The model under review builds one solid part; all positions refer to its coordinate system, in mm. Face numbers are marked on the shaded views. A direction names the side the tool comes from. Round coordinates to 2 decimals unless told otherwise and drop trailing zeros. Loops run counter-clockwise (first coordinate to the right, second up) from the corner with the lowest first, then second, coordinate; pieces in that order, holes last. Notation, with made-up numbers: M 52.5,7.25 L 88.5,7.25 A9 ccw 88.5,23.25 Z; hole C 19,2.5 d6. An arc over 180 degrees is marked long. Return JSON: item names as keys, results as strings. Group by question number.
Q1. Consider section A-A (y = 4.95). State the section outline as (x, z) points.
Q2. To check wall thickness, follow line 1 along Z through (x, y) = (-1.5, 5.3); line 2 along X through (y, z) = (2.05, -0.5); line 3 along Y through (x, z) = (0.25, -0.5). State the ranges of each line that lie inside material, in increasing order.
Q3. Consider section C-C (z = 0.75). State the section outline as (x, y) points.
Q4. Clearance check with flat-ended pins moving along their axes: pin 1 Ø3 at (x, z) = (0, 0) entering from +Y; pin 2 Ø1 at (x, y) = (-0.5, 5) entering from +Z. State where each tip first meets the part, or that it passes through.
Q5. Consider section B-B (x = -1.25). State the section outline as (y, z) points, and give its area (3 significant figures).
Q6. For the marked faces 1 and 2, list the 3-axis set-ups (+Z, -Z, +X, -X, +Y, -Y) from which the entire face can be reached by the end or side of a thin tool; tool diameter is ignored.
Q7. Consider section D-D (z = 2.75). State the section outline as (x, y) points.
Q8. Draft analysis for pull direction X (two halves, no side actions). For the marked faces 3, 4 and 5, state which applies: pulls with the +X half, pulls with the -X half, needs draft (parallel to the pull), parting line crosses it, or undercut.
from build123d import *

# Parameters (mm, degrees)
BOSS_EXTRUDE1_DEPTH = 6
SKETCH2_W           = 4
SKETCH2_H           = 4
CUT_EXTRUDE1_DEPTH  = 5
FILLET1_R           = 0.25


with BuildPart() as part:
    # Sketch1 → Boss-Extrude1 (new body)
    with BuildSketch(Plane(origin=(0, 0, 0), x_dir=(1, 0, 0), z_dir=(0, 1, 0))):
        Polygon((3.214834695, -1.383776673), (2.8058031, 2.092240179), (-0.409031596, 3.476016852), (-3.214834695, 1.383776673), (-2.8058031, -2.092240179), (0.409031596, -3.476016852), align=None)
    extrude(amount=BOSS_EXTRUDE1_DEPTH)

    # Sketch2 → Cut-Extrude1 (cut)
    with BuildSketch(Plane(origin=(0, 6, 0), x_dir=(1, 0, 0), z_dir=(0, 1, 0))):
        Rectangle(SKETCH2_W, SKETCH2_H)
    extrude(amount=-CUT_EXTRUDE1_DEPTH, mode=Mode.SUBTRACT)

    # Fillet1
    # the kernel refuses this fillet: 0.25 mm, written as the material it takes off along each edge
    with BuildSketch(Plane(origin=(-2, 6, -2), x_dir=(-1, 0, 0), z_dir=(0, 0, 1)), Plane(origin=(2, 6, -2), x_dir=(0, 0, -1), z_dir=(-1, 0, 0)), Plane(origin=(-2, 6, 2), x_dir=(0, 0, 1), z_dir=(1, 0, 0)), Plane(origin=(2, 6, 2), x_dir=(1, 0, 0), z_dir=(0, 0, -1))) as fillet1_piece_1:
        with BuildLine():
            CenterArc((FILLET1_R, FILLET1_R), FILLET1_R, 180, 90)
            Line((0, FILLET1_R), (-FILLET1_R * 0.02, FILLET1_R))
            Line((-FILLET1_R * 0.02, FILLET1_R), (-FILLET1_R * 0.02, -FILLET1_R * 0.02))
            Line((-FILLET1_R * 0.02, -FILLET1_R * 0.02), (FILLET1_R, -FILLET1_R * 0.02))
            Line((FILLET1_R, -FILLET1_R * 0.02), (FILLET1_R, 0))
        make_face()
    extrude(amount=4, mode=Mode.SUBTRACT)
    with BuildSketch(Plane(origin=(2, 6, -2), x_dir=(0, 0, -1), z_dir=(-1, 0, 0))) as fillet1_piece_2a_section:
        with BuildLine():
            CenterArc((FILLET1_R, FILLET1_R), FILLET1_R, 180, 90)
            Line((0, FILLET1_R), (-FILLET1_R * 0.02, FILLET1_R))
            Line((-FILLET1_R * 0.02, FILLET1_R), (-FILLET1_R * 0.02, -FILLET1_R * 0.02))
            Line((-FILLET1_R * 0.02, -FILLET1_R * 0.02), (FILLET1_R, -FILLET1_R * 0.02))
            Line((FILLET1_R, -FILLET1_R * 0.02), (FILLET1_R, 0))
        make_face()
    fillet1_piece_2a = extrude(amount=4.625, mode=Mode.PRIVATE)
    fillet1_piece_2a = split(fillet1_piece_2a, bisect_by=Plane(origin=(-2, 5.943401221, -2.056598779), z_dir=(-1, 0, 0)), keep=Keep.TOP, mode=Mode.PRIVATE)
    with BuildSketch(Plane(origin=(-2, 6, -2.625), x_dir=(-1, 0, 0), z_dir=(0, 0, 1))) as fillet1_piece_2b_section:
        with BuildLine():
            CenterArc((FILLET1_R, FILLET1_R), FILLET1_R, 180, 90)
            Line((0, FILLET1_R), (-FILLET1_R * 0.02, FILLET1_R))
            Line((-FILLET1_R * 0.02, FILLET1_R), (-FILLET1_R * 0.02, -FILLET1_R * 0.02))
            Line((-FILLET1_R * 0.02, -FILLET1_R * 0.02), (FILLET1_R, -FILLET1_R * 0.02))
            Line((FILLET1_R, -FILLET1_R * 0.02), (FILLET1_R, 0))
        make_face()
    fillet1_piece_2b = extrude(amount=4.625, mode=Mode.PRIVATE)
    fillet1_piece_2b = split(fillet1_piece_2b, bisect_by=Plane(origin=(-2.056598779, 5.943401221, -2), z_dir=(0, 0, -1)), keep=Keep.TOP, mode=Mode.PRIVATE)
    fillet1_piece_2 = fillet1_piece_2a & fillet1_piece_2b
    add(fillet1_piece_2, mode=Mode.SUBTRACT)
    with BuildSketch(Plane(origin=(-2.625, 6, 2), x_dir=(0, 0, 1), z_dir=(1, 0, 0))) as fillet1_piece_3a_section:
        with BuildLine():
            CenterArc((FILLET1_R, FILLET1_R), FILLET1_R, 180, 90)
            Line((0, FILLET1_R), (-FILLET1_R * 0.02, FILLET1_R))
            Line((-FILLET1_R * 0.02, FILLET1_R), (-FILLET1_R * 0.02, -FILLET1_R * 0.02))
            Line((-FILLET1_R * 0.02, -FILLET1_R * 0.02), (FILLET1_R, -FILLET1_R * 0.02))
            Line((FILLET1_R, -FILLET1_R * 0.02), (FILLET1_R, 0))
        make_face()
    fillet1_piece_3a = extrude(amount=4.625, mode=Mode.PRIVATE)
    fillet1_piece_3a = split(fillet1_piece_3a, bisect_by=Plane(origin=(-2, 5.943401221, 2.056598779), z_dir=(-1, 0, 0)), keep=Keep.TOP, mode=Mode.PRIVATE)
    with BuildSketch(Plane(origin=(-2, 6, -2), x_dir=(-1, 0, 0), z_dir=(0, 0, 1))) as fillet1_piece_3b_section:
        with BuildLine():
            CenterArc((FILLET1_R, FILLET1_R), FILLET1_R, 180, 90)
            Line((0, FILLET1_R), (-FILLET1_R * 0.02, FILLET1_R))
            Line((-FILLET1_R * 0.02, FILLET1_R), (-FILLET1_R * 0.02, -FILLET1_R * 0.02))
            Line((-FILLET1_R * 0.02, -FILLET1_R * 0.02), (FILLET1_R, -FILLET1_R * 0.02))
            Line((FILLET1_R, -FILLET1_R * 0.02), (FILLET1_R, 0))
        make_face()
    fillet1_piece_3b = extrude(amount=4.625, mode=Mode.PRIVATE)
    fillet1_piece_3b = split(fillet1_piece_3b, bisect_by=Plane(origin=(-2.056598779, 5.943401221, 2), z_dir=(0, 0, 1)), keep=Keep.TOP, mode=Mode.PRIVATE)
    fillet1_piece_3 = fillet1_piece_3a & fillet1_piece_3b
    add(fillet1_piece_3, mode=Mode.SUBTRACT)
    with BuildSketch(Plane(origin=(2, 6, 2), x_dir=(1, 0, 0), z_dir=(0, 0, -1))) as fillet1_piece_4a_section:
        with BuildLine():
            CenterArc((FILLET1_R, FILLET1_R), FILLET1_R, 180, 90)
            Line((0, FILLET1_R), (-FILLET1_R * 0.02, FILLET1_R))
            Line((-FILLET1_R * 0.02, FILLET1_R), (-FILLET1_R * 0.02, -FILLET1_R * 0.02))
            Line((-FILLET1_R * 0.02, -FILLET1_R * 0.02), (FILLET1_R, -FILLET1_R * 0.02))
            Line((FILLET1_R, -FILLET1_R * 0.02), (FILLET1_R, 0))
        make_face()
    fillet1_piece_4a = extrude(amount=4.625, mode=Mode.PRIVATE)
    fillet1_piece_4a = split(fillet1_piece_4a, bisect_by=Plane(origin=(2.056598779, 5.943401221, -2), z_dir=(0, 0, -1)), keep=Keep.TOP, mode=Mode.PRIVATE)
    with BuildSketch(Plane(origin=(2.625, 6, -2), x_dir=(0, 0, -1), z_dir=(-1, 0, 0))) as fillet1_piece_4b_section:
        with BuildLine():
            CenterArc((FILLET1_R, FILLET1_R), FILLET1_R, 180, 90)
            Line((0, FILLET1_R), (-FILLET1_R * 0.02, FILLET1_R))
            Line((-FILLET1_R * 0.02, FILLET1_R), (-FILLET1_R * 0.02, -FILLET1_R * 0.02))
            Line((-FILLET1_R * 0.02, -FILLET1_R * 0.02), (FILLET1_R, -FILLET1_R * 0.02))
            Line((FILLET1_R, -FILLET1_R * 0.02), (FILLET1_R, 0))
        make_face()
    fillet1_piece_4b = extrude(amount=4.625, mode=Mode.PRIVATE)
    fillet1_piece_4b = split(fillet1_piece_4b, bisect_by=Plane(origin=(2, 5.943401221, -2.056598779), z_dir=(1, 0, 0)), keep=Keep.TOP, mode=Mode.PRIVATE)
    fillet1_piece_4 = fillet1_piece_4a & fillet1_piece_4b
    add(fillet1_piece_4, mode=Mode.SUBTRACT)
    with BuildSketch(Plane(origin=(-2, 6, 2), x_dir=(0, 0, 1), z_dir=(1, 0, 0))) as fillet1_piece_5a_section:
        with BuildLine():
            CenterArc((FILLET1_R, FILLET1_R), FILLET1_R, 180, 90)
            Line((0, FILLET1_R), (-FILLET1_R * 0.02, FILLET1_R))
            Line((-FILLET1_R * 0.02, FILLET1_R), (-FILLET1_R * 0.02, -FILLET1_R * 0.02))
            Line((-FILLET1_R * 0.02, -FILLET1_R * 0.02), (FILLET1_R, -FILLET1_R * 0.02))
            Line((FILLET1_R, -FILLET1_R * 0.02), (FILLET1_R, 0))
        make_face()
    fillet1_piece_5a = extrude(amount=4.625, mode=Mode.PRIVATE)
    fillet1_piece_5a = split(fillet1_piece_5a, bisect_by=Plane(origin=(2, 5.943401221, 2.056598779), z_dir=(1, 0, 0)), keep=Keep.TOP, mode=Mode.PRIVATE)
    with BuildSketch(Plane(origin=(2, 6, 2.625), x_dir=(1, 0, 0), z_dir=(0, 0, -1))) as fillet1_piece_5b_section:
        with BuildLine():
            CenterArc((FILLET1_R, FILLET1_R), FILLET1_R, 180, 90)
            Line((0, FILLET1_R), (-FILLET1_R * 0.02, FILLET1_R))
            Line((-FILLET1_R * 0.02, FILLET1_R), (-FILLET1_R * 0.02, -FILLET1_R * 0.02))
            Line((-FILLET1_R * 0.02, -FILLET1_R * 0.02), (FILLET1_R, -FILLET1_R * 0.02))
            Line((FILLET1_R, -FILLET1_R * 0.02), (FILLET1_R, 0))
        make_face()
    fillet1_piece_5b = extrude(amount=4.625, mode=Mode.PRIVATE)
    fillet1_piece_5b = split(fillet1_piece_5b, bisect_by=Plane(origin=(2.056598779, 5.943401221, 2), z_dir=(0, 0, 1)), keep=Keep.TOP, mode=Mode.PRIVATE)
    fillet1_piece_5 = fillet1_piece_5a & fillet1_piece_5b
    add(fillet1_piece_5, mode=Mode.SUBTRACT)


solid = part.part
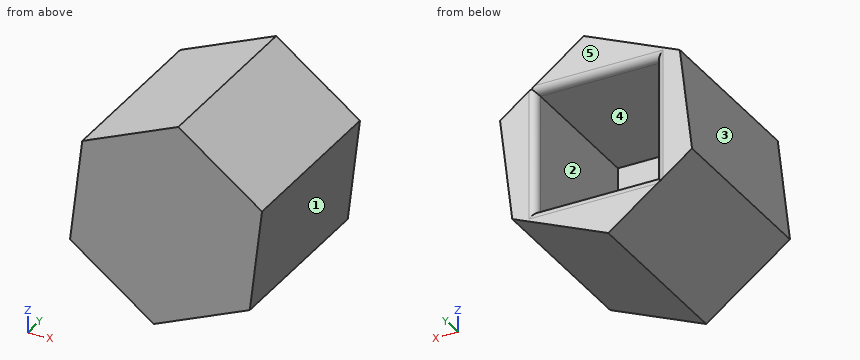
Values:
{
 "1": {"outline": "M -3.21,-1.38 L -0.41,-3.48 L 2.81,-2.09 L 3.21,1.38 L 0.41,3.48 L -2.81,2.09 Z; hole M -2,-2 L 2,-2 L 2,2 L -2,2 Z"},
 "2": {"line 1": "z = -2.66 to -2, 2 to 2.65", "line 2": "x = -3.11 to -2, 2 to 2.99", "line 3": "y = 0 to 1"},
 "3": {"outline": "M -2.96,0 L 3.14,0 L 3.14,6 L 2.25,6 A0.25 ccw 2,5.75 L 2,1 L -2,1 L -2,5.75 A0.25 ccw -2.25,6 L -2.96,6 Z"},
 "4": {"pin 1": "stops at y = 1", "pin 2": "stops at z = 3.3"},
 "5": {"outline": "M 0,-2.85 L 6,-2.85 L 6,-2.25 A0.25 ccw 5.75,-2 L 1,-2 L 1,2 L 5.75,2 A0.25 ccw 6,2.25 L 6,2.76 L 0,2.76 Z", "area": "13.6 mm2"},
 "6": {"face 1": "-Z, +X, +Y, -Y", "face 2": "+Y"},
 "7": {"outline": "M -1.28,0 L 1.38,0 L 1.38,6 L -1.28,6 Z"},
 "8": {"face 3": "pulls with the -X half", "face 4": "undercut", "face 5": "needs draft"}
}
